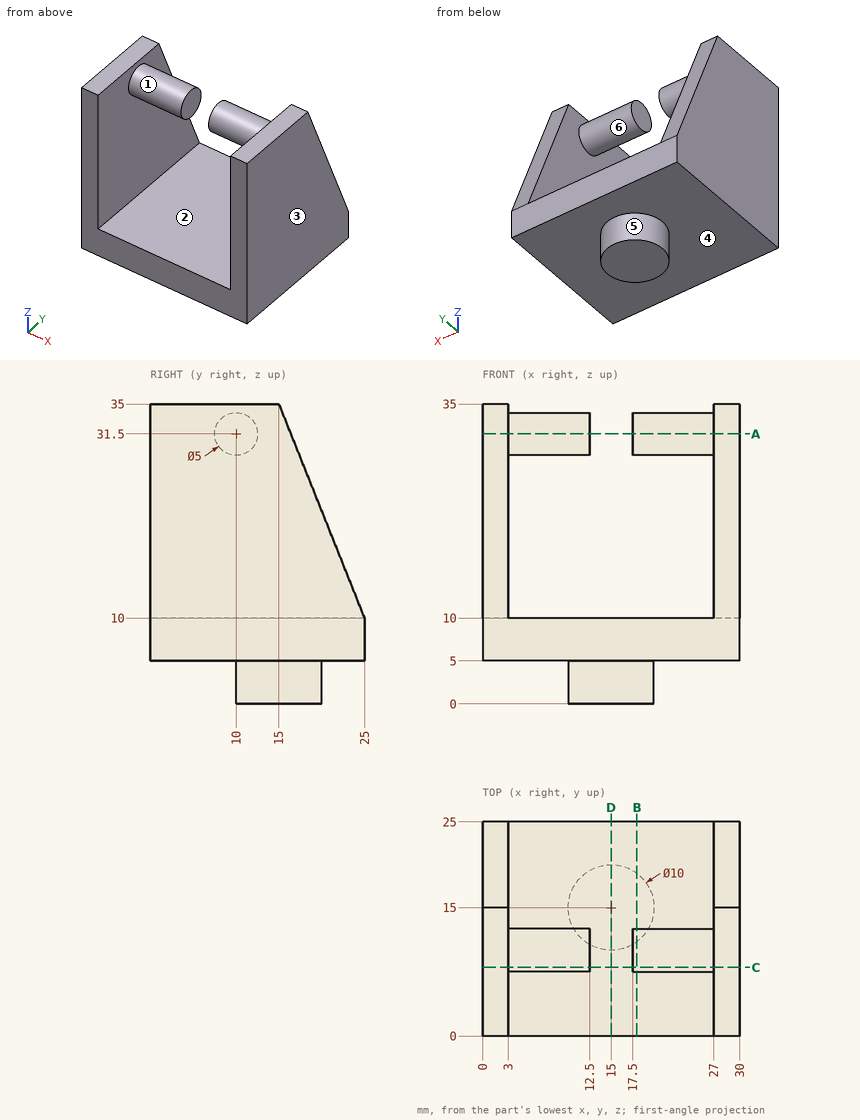
Verification items for this drawing (mm, ordinates from the low corner). A direction names the side the tool comes from. Round coordinates to 2 decimals unless told otherwise and drop trailing zeros. Loops run counter-clockwise (first coordinate to the right, second up) from the corner with the lowest first, then second, coordinate; pieces in that order, holes last. Notation, with made-up numbers: (-4.75, 85.25) - (34.25, 85.25) arc R15 ccw to (34.25, 111.25) - close; hole circle Ø8 at (-25, 32.25). An arc over 180 degrees is marked (long way). Write item = value, one per line.
Q1. Sectioned sample at B-B on x = 18. Record the boundary of the cut face in (y, z), plus the area to 3 significant figures.
Here are the results:
outline = (0, 5) - (11, 5) - (11, 0) - (19, 0) - (19, 5) - (25, 5) - (25, 10) - (0, 10) - close; circle Ø5 at (10, 31.5)
area = 185 mm^2
Q2. Sectioned sample at C-C on y = 8. Record the boundary of the cut face in (x, z), plus the area to 3 significant figures.
Here are the results:
outline = (0, 5) - (30, 5) - (30, 35) - (27, 35) - (27, 33) - (17.5, 33) - (17.5, 30) - (27, 30) - (27, 10) - (3, 10) - (3, 30) - (12.5, 30) - (12.5, 33) - (3, 33) - (3, 35) - (0, 35) - close
area = 357 mm^2
Q3. Material ranges on L1, parallel to X at y = 2.5, z = 21.5; L2, parallel to Z at x = 4, y = 19.5; L3, parallel to Z at x = 16.25, y = 14, recorded low to high.
Here are the results:
L1 = 0 to 3, 27 to 30
L2 = 5 to 10
L3 = 0 to 10
Q4. Sectioned sample at A-A on z = 31.5. Record the boundary of the cut face in (x, y).
Here are the results:
outline = (0, 0) - (3, 0) - (3, 7.5) - (12.5, 7.5) - (12.5, 12.5) - (3, 12.5) - (3, 16.4) - (0, 16.4) - close; (17.5, 7.5) - (27, 7.5) - (27, 0) - (30, 0) - (30, 16.4) - (27, 16.4) - (27, 12.5) - (17.5, 12.5) - close
Q5. Tool access check on the marked faces 1, 2 and 3. Record the directions out of +Z, -Z, +X, -X, +Y, -Y that give a thin tool (end or side, any length) a straight path to the whole face; none if there is none.
Here are the results:
face_1 = none
face_2 = +Y, -Y
face_3 = +Z, -Z, +X, +Y, -Y
Q6. Sectioned sample at D-D on x = 15. Record the boundary of the cut face in (y, z), plus the area to 3 significant figures.
Here are the results:
outline = (0, 5) - (10, 5) - (10, 0) - (20, 0) - (20, 5) - (25, 5) - (25, 10) - (0, 10) - close
area = 175 mm^2
Q7. Mould release check, pull along Z, two halves, no side actions. Record for the marked faces 4, 5 and 6: +Z half, -Z half, draft (parallel to the pull), parting line (faces both ways), or undercut.
Here are the results:
face_4 = -Z half
face_5 = draft
face_6 = undercut
Q8. Depth check by flat-ended pin: pin 1 (10 mm diameter, centred on x = 20.5, y = 18.5, fed in from -Z); pin 2 (12 mm diameter, centred on x = 17, y = 10.5, fed in from +Z). Enter the tip coordinate at first touch or a pass-through.
Here are the results:
pin_1 = 0
pin_2 = 34
